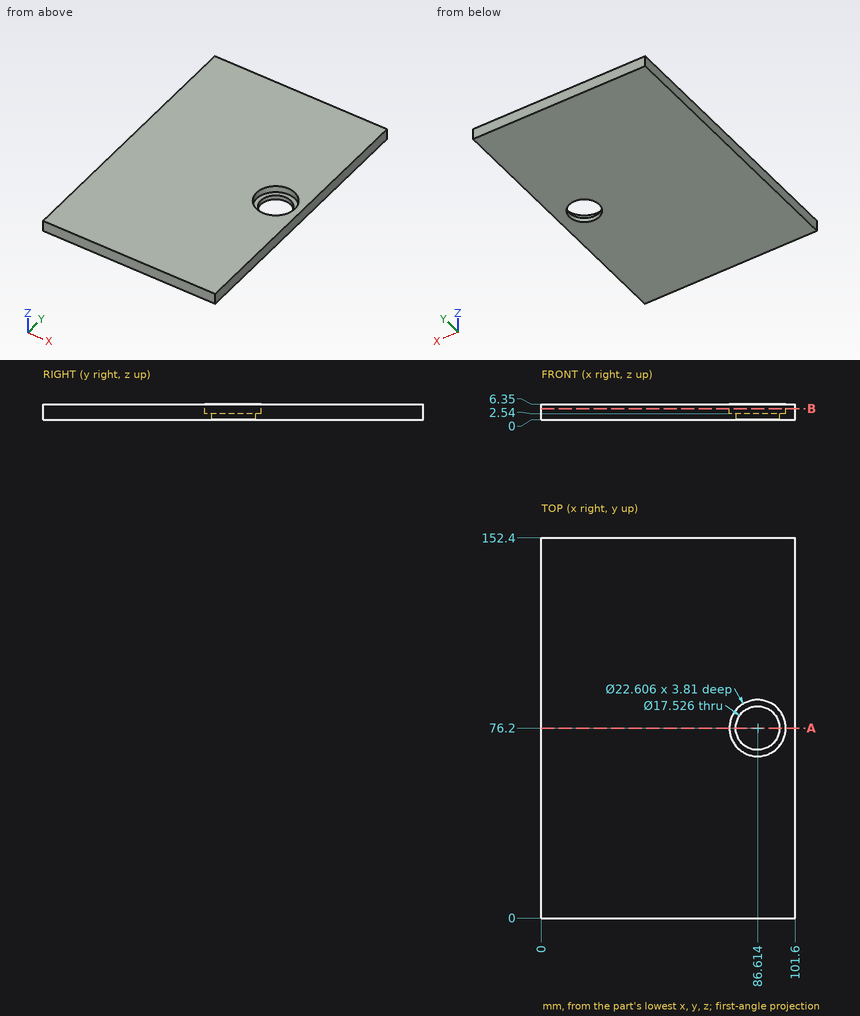
For this review, use the dimensioned drawing (mm, ordinates from the lowest corner) and the shaded views. Coordinates: 2 decimals unless noted, no trailing zeros. Loops run counter-clockwise (first coordinate to the right, second up) from the corner with the lowest first, then second, coordinate; pieces in that order, holes last. Notation, with made-up numbers: (74.25, 39.5) - (92.25, 39.5) arc R13 ccw to (92.25, 43.5) - close; hole circle Ø5 at (-26, -36.75). An arc over 180 degrees is marked (long way). Use CSV: the item, a comma, the result in double quotes. Start each with the question number.
1) Wall thickness on L1, parallel to Y at x = 86, z = 4; L2, parallel to Y at x = 82.5, z = 2.25; L3, parallel to X at y = 77.5, z = 4: over which ranges is each line inside the solid? List them lowest first. Write a range as from..to.
2) Consider section A-A on y = 76.2. Write out the cut boundary in (x, z), then the cut area to 3 significant figures.
3) Consider section B-B on z = 4.5. Write out the cut boundary in (x, y), then the cut area to 3 significant figures.
4) For pin 1 Ø11.5 at (x, y) = (81.5, 75) entering from +Z, flat-tipped, find the tip position at first contact; note if it passes through.
Geometry says:
1,L1,"0..64.91, 87.49..152.4"
1,L2,"0..68.46, 83.94..152.4"
1,L3,"0..75.39, 97.84..101.6"
2,outline,"(0, 0) - (77.85, 0) - (77.85, 2.54) - (75.31, 2.54) - (75.31, 6.35) - (0, 6.35) - close; (95.38, 0) - (101.6, 0) - (101.6, 6.35) - (97.92, 6.35) - (97.92, 2.54) - (95.38, 2.54) - close"
2,area,"515 mm^2"
3,outline,"(0, 0) - (101.6, 0) - (101.6, 152.4) - (0, 152.4) - close; hole circle Ø22.61 at (86.61, 76.2)"
3,area,"15,100 mm^2"
4,pin 1,"z = 2.54"
